Design review of the part built by this model. Coordinates are the model's own, in mm. Face numbers are marked on the shaded views. A direction names the side the tool comes from. Coordinates: 2 decimals unless noted, no trailing zeros. Loops run counter-clockwise (first coordinate to the right, second up) from the corner with the lowest first, then second, coordinate; pieces in that order, holes last. Notation, with made-up numbers: (49.25, 52.25) -> (108.25, 52.25) arc R18 cw to (108.25, 76.25) -> close; hole circle Ø6 at (50, -14.5). An arc over 180 degrees is marked (long way). Answer in a Markdown table with one row per item.
```python
from build123d import *

# Parameters (mm, degrees)
EXTRUSI_N_HEX_PROFILE_DEPTH = 19.7866


with BuildPart() as part:
    # Croquis2 → Extrusi_n Hex Profile (new, symmetric)
    with BuildSketch(Plane.XY):
        Polygon((3.666174209, -6.35), (7.332348419, 0), (3.666174209, 6.35), (-3.666174209, 6.35), (-7.332348419, 0), (-3.666174209, -6.35), align=None)
    extrude(amount=EXTRUSI_N_HEX_PROFILE_DEPTH, both=True)

    # Croquis10 → Round End 1 (revolve, cut)
    with BuildSketch(Plane(origin=(0, 0, 0), x_dir=(1, 0, 0), z_dir=(0, 1, 0)), mode=Mode.PRIVATE) as round_end_1_sk:
        Polygon((-3.96875, -19.7866), (-4.7625, -18.99285), (-4.7625, -12.6492), (-9.525, -12.6492), (-9.525, -19.7866), align=None)
    revolve(round_end_1_sk.sketch.rotate(Axis((0, 0, 19.7866), (0, 0, -1)), 180), axis=Axis((0, 0, 19.7866), (0, 0, -1)), mode=Mode.SUBTRACT)

    # Croquis12 → Round End 2 (revolve, cut)
    with BuildSketch(Plane.XZ):
        Polygon((-3.96875, -19.7866), (-4.7625, -18.99285), (-4.7625, -12.6492), (-9.525, -12.6492), (-9.525, -19.7866), align=None)
    revolve(axis=Axis((0, 0, -19.7866), (0, 0, 1)), mode=Mode.SUBTRACT)


solid = part.part
```
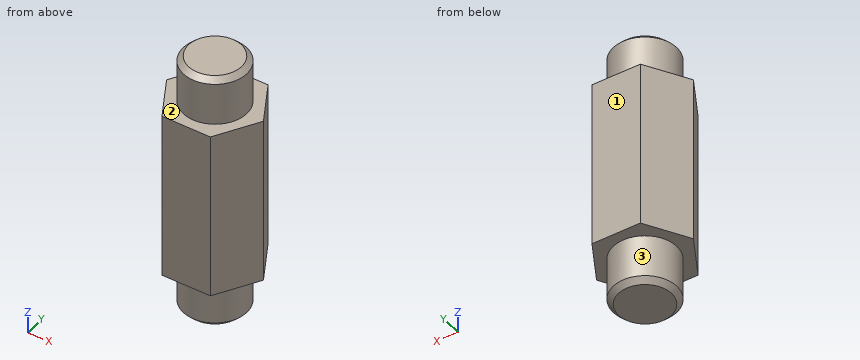
(1) Take a section at D-D on x = -6. Give the boundary of the cut face in (y, z), and give its area (3 significant figures).
Evaluation:
| item | result |
|---|---|
| outline | (-2.31, -12.65) -> (2.31, -12.65) -> (2.31, 12.65) -> (-2.31, 12.65) -> close |
| area | 117 mm² |
(2) To check wall thickness, follow probe 1 along Z at (x, y) = (5.75, 1.25); probe 2 along X at (y, z) = (0.25, 17.5); probe 3 along X at (y, z) = (-0.75, 11). State the ranges of each line that lie inside material, in increasing order.
Evaluation:
| item | result |
|---|---|
| probe 1 | z = -12.65 to 12.65 |
| probe 2 | x = -4.76 to 4.76 |
| probe 3 | x = -6.9 to 6.9 |
(3) Take a section at C-C on z = -14. Give the boundary of the cut face in (x, y) (1 decimal).
Evaluation:
| item | result |
|---|---|
| outline | circle Ø9.5 at (0, 0) |
(4) Take a section at B-B on z = -7. Give the boundary of the cut face in (x, y).
Evaluation:
| item | result |
|---|---|
| outline | (-7.33, 0) -> (-3.67, -6.35) -> (3.67, -6.35) -> (7.33, 0) -> (3.67, 6.35) -> (-3.67, 6.35) -> close |
(5) For pin 1 (5 mm diameter, centred on y = 4, z = 13, fed in from -X); pin 2 (2 mm diameter, centred on y = 0.5, z = 11.5, fed in from +X); pin 3 (1.5 mm diameter, centred on x = 5, y = -3.5, fed in from +Z), all flat-tipped, find the tip position at first contact; note any pin that passes through.
Evaluation:
| item | result |
|---|---|
| pin 1 | stops at x = -6.45 |
| pin 2 | stops at x = 7.33 |
| pin 3 | stops at z = 12.65 |
(6) Tool access review of the marked faces 1, 2 and 3: name each direction out of +Z, -Z, +X, -X, +Y, -Y from which nothing blocks a thin tool from reaching the whole face with its end or side.
Evaluation:
| item | result |
|---|---|
| face 1 | +Z, -Z, +X, -X, +Y |
| face 2 | +Z |
| face 3 | -Z |
(7) Take a section at A-A on x = 0. Give the boundary of the cut face in (y, z).
Evaluation:
| item | result |
|---|---|
| outline | (-6.35, -12.65) -> (-4.76, -12.65) -> (-4.76, -18.99) -> (-3.97, -19.79) -> (3.97, -19.79) -> (4.76, -18.99) -> (4.76, -12.65) -> (6.35, -12.65) -> (6.35, 12.65) -> (4.76, 12.65) -> (4.76, 18.99) -> (3.97, 19.79) -> (-3.97, 19.79) -> (-4.76, 18.99) -> (-4.76, 12.65) -> (-6.35, 12.65) -> close |
